Answer from the drawing. Dimensions are ordinates in mm from the lowest x, y and z of the part. Coordinates: 2 decimals unless noted, no trailing zeros. Write each loop counter-clockwise with the first axis right and the second up, starting at its lowest first coordinate (ties: lowest second). Pieces come first, ordered by that corner, then holes. Notation, with made-up numbers: (29.5, 13) - (40.5, 13) arc R12 cw to (40.5, 29) - close; hole circle Ø5 at (-21.5, 73). An arc over 180 degrees is marked (long way). Answer as a JSON object with one key per item and string values. Group by question number.
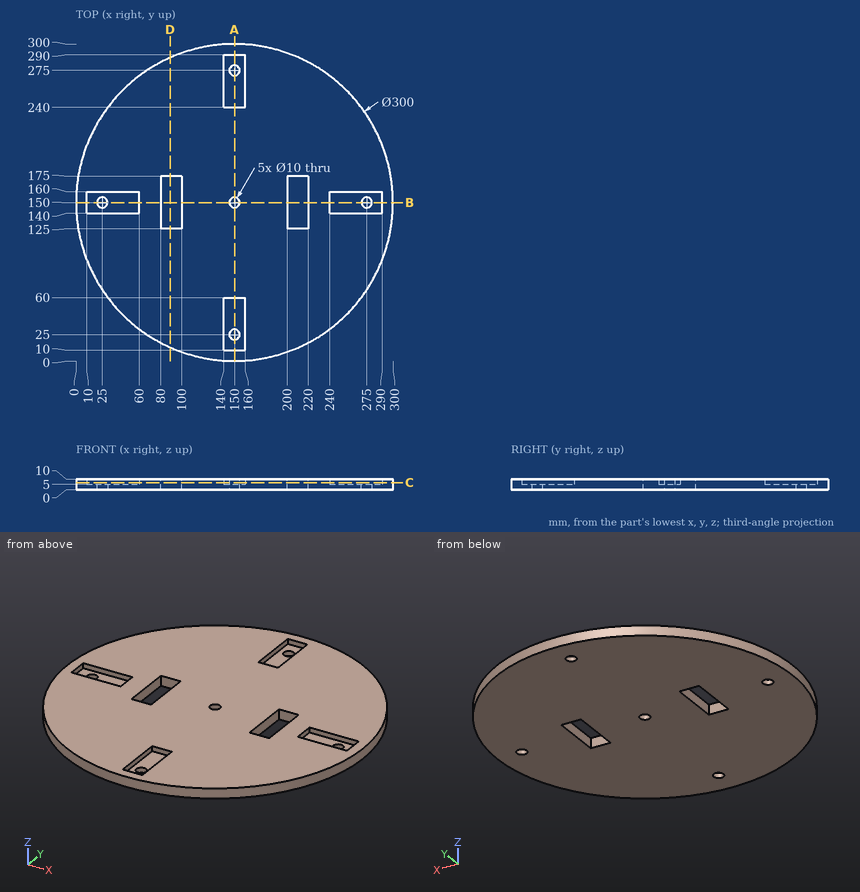
Q1. Consider L1, parallel to Y at x = 150, z = 2.3; L2, parallel to X at y = 171, z = 6; L3, parallel to X at y = 146, z = 1.5. Determine where each line is inside the solid, lowest interval first. Write a range as from..to.
Q2. Section D-D on x = 89 is taken. Determine the outline of the cut face in (y, z).
Q3. Section B-B on y = 150 is taken. Count the separate pieces of the cut face and the enclosed holes in it, plus the area to 3 significant figures.
Q4. Flat-ended cylindrical pins translate along their axes: pin 1 Ø3 at (x, z) = (216.5, 1.5) entering from +Y; pin 2 Ø16 at (x, y) = (150, 25) entering from +Z; pin 3 Ø1 at (x, z) = (196, 1) entering from +Y; pin 4 Ø12 at (x, y) = (119.5, 41.5) entering from -Z. Find the tip coordinate at first contact, or state that the pin passes through.
Q5. Section A-A on x = 150 is taken. Determine the outline of the cut face in (y, z), plus the area to 3 significant figures.
Q6. Section C-C on z = 6.5 is taken. Determine the outline of the cut face in (x, y), plus the area to 3 significant figures.
Numbers:
{
 "1": {"L1": "y = 0..20, 30..145, 155..270, 280..300", "L2": "x = 1.48..80, 100..200, 220..298.52", "L3": "x = 0.05..22, 28..80, 100..147, 153..200, 220..272, 278..299.95"},
 "2": {"outline": "(12.96, 0) - (125, 0) - (125, 10) - (12.96, 10) - close; (175, 0) - (287.04, 0) - (287.04, 10) - (175, 10) - close"},
 "3": {"separate pieces": "6", "enclosed holes": "0", "area": "1,900 mm²"},
 "4": {"pin 1": "stops at y = 285.19", "pin 2": "stops at z = 5", "pin 3": "stops at y = 292.93", "pin 4": "stops at z = 0"},
 "5": {"outline": "(0, 0) - (20, 0) - (20, 5) - (10, 5) - (10, 10) - (0, 10) - close; (30, 0) - (145, 0) - (145, 10) - (60, 10) - (60, 5) - (30, 5) - close; (155, 0) - (270, 0) - (270, 5) - (240, 5) - (240, 10) - (155, 10) - close; (280, 0) - (300, 0) - (300, 10) - (290, 10) - (290, 5) - (280, 5) - close", "area": "2,300 mm²"},
 "6": {"outline": "circle Ø300 at (150, 150); hole (10, 140) - (60, 140) - (60, 160) - (10, 160) - close; hole (80, 125) - (100, 125) - (100, 175) - (80, 175) - close; hole (140, 10) - (160, 10) - (160, 60) - (140, 60) - close; hole (140, 240) - (160, 240) - (160, 290) - (140, 290) - close; hole circle Ø10 at (150, 150); hole (200, 125) - (220, 125) - (220, 175) - (200, 175) - close; hole (240, 140) - (290, 140) - (290, 160) - (240, 160) - close", "area": "64,600 mm²"}
}
